```python
from build123d import *

# Parameters (mm, degrees)
SKETCH1_W           = 34
SKETCH1_H           = 34
BOSS_EXTRUDE1_DEPTH = 3
SKETCH2_W           = 12.5
SKETCH2_H           = 5
CUT_EXTRUDE1_DEPTH  = 49.176757882
BOSS_EXTRUDE2_DEPTH = 5
SKETCH3_R           = 1.4
BOSS_EXTRUDE3_DEPTH = 8
SKETCH33_W          = 15
SKETCH33_H          = 5
BOSS_EXTRUDE4_DEPTH = 5
BOSS_EXTRUDE6_DEPTH = 15
SKETCH36_W          = 24
SKETCH36_H          = 13
CUT_EXTRUDE2_DEPTH  = 19.5
BOSS_EXTRUDE7_DEPTH = 5
SKETCH39_R          = 1.5
CUT_EXTRUDE3_DEPTH  = 61.897668661


with BuildPart() as part:
    # Sketch1 → Boss-Extrude1 (new body)
    with BuildSketch(Plane.XY):
        with Locations((17, -17)):
            Rectangle(SKETCH1_W, SKETCH1_H)
    extrude(amount=BOSS_EXTRUDE1_DEPTH)

    # Sketch2 → Cut-Extrude1 (cut, through all)
    with BuildSketch(Plane(origin=(0, 0, 0), x_dir=(-1, 0, 0), z_dir=(0, 0, -1))):
        with Locations((-17, -2.5)):
            Rectangle(SKETCH2_W, SKETCH2_H)
        with Locations((-17, -31.5)):
            Rectangle(SKETCH2_W, SKETCH2_H)
    extrude(amount=-CUT_EXTRUDE1_DEPTH, mode=Mode.SUBTRACT)

    # Sketch25 → Boss-Extrude2 (add)
    with BuildSketch(Plane(origin=(34, 0, 0), x_dir=(0, 0, -1), z_dir=(1, 0, 0))):
        Polygon((-3, -17), (-3, -14.5), (12, -14.5), (12, -19.5), (-3, -19.5), align=None)
    extrude(amount=BOSS_EXTRUDE2_DEPTH)

    # Sketch3 → Boss-Extrude3 (add)
    with BuildSketch(Plane(origin=(0, 0, 0), x_dir=(-1, 0, 0), z_dir=(0, 0, -1))):
        with Locations((-29.75, -4.25)):
            Circle(SKETCH3_R)
        with Locations(Location((-4.25, -4.25, 0), (0, 0, 180))):
            Circle(SKETCH3_R)
        with Locations((-4.25, -29.75)):
            Circle(SKETCH3_R)
        with Locations(Location((-29.75, -29.75, 0), (0, 0, 180))):
            Circle(SKETCH3_R)
    extrude(amount=-BOSS_EXTRUDE3_DEPTH)

    # Sketch33 → Boss-Extrude4 (add)
    with BuildSketch(Plane.ZY):
        with Locations((-4.5, -17)):
            Rectangle(SKETCH33_W, SKETCH33_H)
    extrude(amount=BOSS_EXTRUDE4_DEPTH)

    # Sketch35 → Boss-Extrude6 (add)
    with BuildSketch(Plane(origin=(0, 0, -12), x_dir=(-1, 0, 0), z_dir=(0, 0, -1))):
        Polygon((-39, -17), (-39, 3.277699473), (5, 3.277699473), (5, -17), (5, -34.025954319), (-39, -34.025954319), align=None)
    extrude(amount=BOSS_EXTRUDE6_DEPTH)

    # Sketch36 → Cut-Extrude2 (cut)
    with BuildSketch(Plane(origin=(0, 3.277699473, 0), x_dir=(1, 0, 0), z_dir=(0, 1, 0))):
        with Locations((17, 19.5)):
            Rectangle(SKETCH36_W, SKETCH36_H)
    extrude(amount=-CUT_EXTRUDE2_DEPTH, mode=Mode.SUBTRACT)

    # Sketch38 → Boss-Extrude7 (add)
    with BuildSketch(Plane(origin=(0, -34.025954319, 0), x_dir=(-1, 0, 0), z_dir=(0, -1, 0))):
        Polygon((10, 21.910063987), (5, 21.910063987), (5, 17.089936013), (10, 17.089936013), (10, 19.410063987), (10, 19.589936013), align=None)
        Polygon((-39, 17.089936013), (-39, 21.910063987), (-44, 21.910063987), (-44, 19.589936013), (-44, 19.410063987), (-44, 17.089936013), align=None)
    extrude(amount=-BOSS_EXTRUDE7_DEPTH)

    # Sketch39 → Cut-Extrude3 (cut, through all)
    with BuildSketch(Plane(origin=(0, -29.025954319, 0), x_dir=(1, 0, 0), z_dir=(0, 1, 0))):
        with Locations(Location((-7.5, 19.5, 0), (0, 0, 270))):
            Circle(SKETCH39_R)
        with Locations(Location((41.5, 19.5, 0), (0, 0, 270))):
            Circle(SKETCH39_R)
    extrude(amount=-CUT_EXTRUDE3_DEPTH, mode=Mode.SUBTRACT)


solid = part.part
```
For this review, take the finished solid that the model builds, in its own axes (mm). A direction names the side the tool comes from. Give positions to 0.01 mm unless a question says otherwise; leave off trailing zeros. Write each loop counter-clockwise with the first axis right and the second up, starting at its lowest first coordinate (ties: lowest second). Pieces come first, ordered by that corner, then holes.
Item 1: Take a section at D-D (z = -7.5). Give the boundary of the cut face in (x, y).
Item 2: Machinability: for faces 1 (the face through (17, -6, -26)), 2 (the face through (23.25, -3, 1)), 3 (the face through (34, -17, -6)), 4 (the face through (36, -14.5, -4)), 5 (the face through (17, -29, 1)), which of the approach directions +Z, -Z, +X, -X, +Y, -Y give a long, thin tool a straight path to every point of the face, cutting with its end or side? Answer none if there is none.
Item 3: The part is to be moulded in two halves that separate along Z. For faces 6 (the face through (17, -5, 1)), 7 (the face through (17, -17, 3)), 8 (the face through (5, -6, -19)), 9 (the face through (-8.4, -31.5, -20.7)), say which applies: +Z half, -Z half, draft (parallel to the pull), parting line (faces both ways), or undercut.
Item 4: Wall thickness on probe 1 along X at (y, z) = (-32.9, -19.5); probe 2 along Z at (x, y) = (23, -12.5); probe 3 along Z at (x, y) = (22, -23.5): over which ranges is each line inside the solid? List them lowest first.
Item 5: Take a section at A-A (y = -4.25). Give the boundary of the cut face in (x, z).
Item 6: Take a section at C-C (z = -19.5). Give the boundary of the cut face in (x, y), and give its area (3 significant figures).
Item 7: Take a section at B-B (x = -7.5). Give the boundary of the cut face in (y, z).
Item 8: Insertion check: P1, Ø3, axis at x = 19.5, y = -10.5, coming from the +Z side; P2, Ø6.5, axis at y = -4, z = -17.5, coming from the -X side; P3, Ø2.5, axis at x = 26.5, z = 2, coming from the +Y side. Each pin has a flat end and moves straight along its axis. Give the tip position at first contact, or say it passes through.
Established:
1. outline: (-5, -19.5) - (0, -19.5) - (0, -14.5) - (-5, -14.5) - close; (34, -19.5) - (39, -19.5) - (39, -14.5) - (34, -14.5) - close
2. face 1: +Y
2. face 2: +Z, +Y
2. face 3: +Y, -Y
2. face 4: +Z, +X, +Y
2. face 5: +Z, -Y
3. face 6: draft
3. face 7: +Z half
3. face 8: undercut
3. face 9: undercut
4. probe 1: x = -10 to -9, -6 to 40, 43 to 44
4. probe 2: z = -27 to -26, -13 to -12, 0 to 3
4. probe 3: z = -27 to -12, 0 to 3
5. outline: (-5, -27) - (39, -27) - (39, -12) - (-5, -12) - close; (0, 0) - (10.75, 0) - (10.75, 3) - (5.65, 3) - (5.65, 8) - (2.85, 8) - (2.85, 3) - (0, 3) - close; (23.25, 0) - (34, 0) - (34, 3) - (31.15, 3) - (31.15, 8) - (28.35, 8) - (28.35, 3) - (23.25, 3) - close; hole (5, -26) - (29, -26) - (29, -13) - (5, -13) - close
6. outline: (-10, -34.03) - (-9, -34.03) - (-9, -29.03) - (-10, -29.03) - close; (-6, -34.03) - (40, -34.03) - (40, -29.03) - (39, -29.03) - (39, 3.28) - (29, 3.28) - (29, -16.22) - (5, -16.22) - (5, 3.28) - (-5, 3.28) - (-5, -29.03) - (-6, -29.03) - close; (43, -34.03) - (44, -34.03) - (44, -29.03) - (43, -29.03) - close
6. area: 1,190 mm2
7. outline: (-34.03, -21.91) - (-29.03, -21.91) - (-29.03, -21) - (-34.03, -21) - close; (-34.03, -18) - (-29.03, -18) - (-29.03, -17.09) - (-34.03, -17.09) - close
8. P1: stops at z = 3
8. P2: stops at x = -5
8. P3: stops at y = 0
